Input: part model. Units: mm. Frame: model coordinates. A direction names the side the tool comes from. Coordinates: 2 decimals unless noted, no trailing zeros. Loops run counter-clockwise (first coordinate to the right, second up) from the corner with the lowest first, then second, coordinate; pieces in that order, holes last. Notation, with made-up numbers: (21, 29) -> (68, 29) arc R23 cw to (68, 45) -> close; hole circle Ø1 at (17.25, 60.5). An arc over 180 degrees is marked (long way). Put each result on its own line as item: value. Start each with the question number.
1) Contact query for flat-ended pins moving along their axis: P1, Ø10, axis at x = -4, y = -31, coming from the +Z side; P2, Ø8, axis at x = -5, y = -2.5, coming from the +Z side; P3, Ø8, axis at x = 0.5, z = -2, coming from the +Y side. Output: stop coordinate, or through.
2) Cut plane A-A (y = -22.5). Return the cut outline in (x, z).
3) Cut plane B-B (z = 49). Return the cut outline in (x, y).
4) Material intervals for L1, parallel to Y at x = 5.75, z = 6; L2, parallel to Z at x = -0.5, y = 10.5; L3, parallel to Z at x = 0, y = -4, sorted ascending.
5) Pull-direction query (Z, two-part tool) for faces 3 (the flat face through (0, 0, -8)), 4 (the flat face through (0, -45.1, 0)); classes: pulls with the +Z half, pulls with the -Z half, needs draft (parallel to the pull), parting line crosses it, or undercut.
6) Set-up query: faces 1 (the flat face through (0, 15, 65)), 2 (the cylindrical face through (0.2, -2.85, 39.27)). Return all of +Z, -Z, +X, -X, +Y, -Y with unobstructed straight access to the full face (end or side cutting, diameter ignored); none if empty.
from build123d import *

# Parameters (mm, degrees)
F0_R        = 12.55
F1_DEPTH    = 45.1
F2_R        = 7.5
F3_DEPTH    = 3
F6_DEPTH    = 75
F7_T2_ANGLE = 359.64
F9_R        = 6.25
F10_DEPTH   = 25


# Not quite as in the source:
# - a fillet or chamfer that OpenCascade refuses, or shapes differently, is made with other operations: its cross-section is extruded or revolved along the edge and cut away or added


with BuildPart() as f1:
    # F0 (on Front) → F1 (new body)
    with BuildSketch(Plane.XZ):
        Circle(F0_R)
    extrude(amount=F1_DEPTH)

    # F2 (on Front) → F3 (join)
    with BuildSketch(Plane.XZ):
        Circle(F2_R)
    extrude(amount=-F3_DEPTH)

    # F4: fillet of radius 10 on 1 edges, made by hand

    # F4_s1 → F4_t2 (revolve, cut)
    with BuildSketch(Plane.XY):
        with BuildLine():
            ThreePointArc((7.5, 0), (4.2315549177, 2.2195444573), (0.3585715715, 3))
            Line((0.3585715715, 3), (7.5, 3))
            Line((7.5, 3), (7.5, 0))
        make_face()
    revolve(axis=Axis((0, 3, 0), (0, -1, 0)), mode=Mode.SUBTRACT)

    # F5 (on Top) → F6 (join)
    with BuildSketch(Plane.XY):
        with BuildLine():
            Line((-12.4928209826, -12.5774559094), (12.6060726016, -12.3417848491))
            ThreePointArc((12.6060726016, -12.3417848491), (-0.0335977446, -2.8508403226), (-12.4928209826, -12.5774559094))
        make_face()
    extrude(amount=F6_DEPTH)

    # F7: fillet of radius 10 on 1 edges, made by hand

    # F7_s1 → F7_t2 (revolve, cut)
    with BuildSketch(Plane(origin=(-0.1101500857, -0.0013803647, 0), x_dir=(0, 0, 1), z_dir=(-0.9999214878, -0.0125306879, 0))):
        with BuildLine():
            ThreePointArc((65, -28.8501313418), (72.0710678119, -25.9211991536), (75, -18.8501313418))
            Line((75, -18.8501313418), (75, -28.8501313418))
            Line((75, -28.8501313418), (65, -28.8501313418))
        make_face()
    revolve(axis=Axis((0.0884629639, -15.8502672786, 75), (0, 0, 1)), revolution_arc=F7_T2_ANGLE, mode=Mode.SUBTRACT)

    # F9 (on offset) → F10 (join)
    with BuildSketch(Plane.XZ.offset(10)):
        with Locations((-0.0335977446, 65)):
            Circle(F9_R)
    extrude(amount=-F10_DEPTH)


solid = f1.part
Results found:
1. P1: stops at z = 12.55
1. P2: stops at z = 71.85
1. P3: stops at y = 3
2. outline: circle Ø25.1 at (0, 0)
3. outline: (-12.49, -12.58) -> (12.61, -12.34) arc R13 ccw to start
4. L1: y = -45.1 to 0
4. L2: z = 58.77 to 71.23
4. L3: z = -12.55 to 71.25
5. face 3: undercut
5. face 4: needs draft
6. face 1: +Z, -Z, +X, -X, +Y
6. face 2: +Y
